```python
from build123d import *

# Parameters (mm, degrees)
KEY1SKETCH_R       = 6.5
KEYPADPAD_DEPTH    = 5
KEY2SKETCH_R       = 6.5
KEYPADPAD001_DEPTH = 5
PIN1SKETCH001_R    = 2
PIN1POCKET_DEPTH   = 10
PIN2SKETCH001_R    = 2
PIN2POCKET_DEPTH   = 10


with BuildPart() as part:
    # key1Sketch → keyPadPad (new body)
    with BuildSketch(Plane.XY):
        with Locations((2, 0)):
            Circle(KEY1SKETCH_R)
    extrude(amount=KEYPADPAD_DEPTH)

    # key2Sketch → keyPadPad001 (join)
    with BuildSketch(Plane.XY.offset(5)):
        with Locations((-2, 0)):
            Circle(KEY2SKETCH_R)
    extrude(amount=KEYPADPAD001_DEPTH)

    # Pin1Sketch001 → Pin1Pocket (cut)
    with BuildSketch(Plane.XY.offset(5)):
        with Locations((1.75, 0)):
            Circle(PIN1SKETCH001_R)
    extrude(amount=-PIN1POCKET_DEPTH, mode=Mode.SUBTRACT)

    # Pin2Sketch001 → Pin2Pocket (cut)
    with BuildSketch(Plane.XY.offset(5)):
        with Locations((3.5, 0)):
            Circle(PIN2SKETCH001_R)
    extrude(amount=-PIN2POCKET_DEPTH, mode=Mode.SUBTRACT)


with BuildPart() as part_1:
    # eccentricKey placement: moved
    add(part.part.moved(Location((0, 0, 10))))


solid = part_1.part
```
The model under review builds one solid part; all positions refer to its coordinate system, in mm. A direction names the side the tool comes from. Round coordinates to 2 decimals unless told otherwise and drop trailing zeros. Order: outer loops, then holes, each group sorted by start corner. A loop starts at its lowest first (then second) coordinate and runs counter-clockwise, first axis right, second up. Notation, with made-up numbers: (87, 58) -> (124, 58) arc R16 cw to (124, 78) -> close; hole circle Ø9 at (31.5, 18.25). An arc over 180 degrees is marked (long way). One line per item, written item: value. Start each with the question number.
Q1. Take a section at A-A (y = 0). Write out the cut boundary in (x, z), and give its area (3 significant figures).
Q2. Machinability: for faces 4 (the face through (6, 0, 15)), 5 (the face through (-2, 0, 20)), 6 (the face through (0.591, -6.345, 12.465)), which of the approach directions +Z, -Z, +X, -X, +Y, -Y give a long, thin tool a straight path to every point of the face, cutting with its end or side? Answer none if there is none.
Q3. Take a section at C-C (x = -2). Write out the cut boundary in (y, z).
Q4. Clearance check with flat-ended pins moving along their axes: pin 1 Ø1 at (y, z) = (-1.5, 13) entering from -X; pin 2 Ø1.5 at (y, z) = (-5, 12) entering from +X; pin 3 Ø1 at (x, y) = (6.5, 3.5) entering from +Z. State where each tip first meets the part, or that it passes through.
Q5. Take a section at D-D (z = 16.75). Write out the cut boundary in (x, y).
Q6. Wall thickness on line 1 (Y direction, x = 1.75, z = 13.3); line 2 (Z direction, x = 7.5, y = 1.5); line 3 (Y direction, x = 3.5, z = 12.75): over which ranges is each line inside the solid? List them lowest first.
Q7. Take a section at B-B (y = -2.5). Write out the cut boundary in (x, z).
Q8. Mouldability with a two-part tool opening along X and no side actions: class faces 1 (the face through (0.999, -5.767, 17.465)), 2 (the face through (-5, 0, 15)), 3 (the face through (-0.25, 0.06, 12.54)) as released by +X, released by -X, zero draft, split by the parting line, or undercut.
Reported:
1. outline: (-8.5, 15) -> (-4.5, 15) -> (-4.5, 10) -> (-0.25, 10) -> (-0.25, 15) -> (4.5, 15) -> (4.5, 20) -> (-8.5, 20) -> close; (5.5, 10) -> (8.5, 10) -> (8.5, 15) -> (5.5, 15) -> close
1. area: 101 mm2
2. face 4: +Z, +X
2. face 5: +Z, +X, -X, +Y, -Y
2. face 6: -Z
3. outline: (-6.5, 15) -> (-5.12, 15) -> (-5.12, 10) -> (5.12, 10) -> (5.12, 15) -> (6.5, 15) -> (6.5, 20) -> (-6.5, 20) -> close
4. pin 1: stops at x = -4.42
4. pin 2: stops at x = 6.92
4. pin 3: stops at z = 15
5. outline: circle Ø13 at (-2, 0)
6. line 1: y = -6.5 to -2, 2 to 6.5
6. line 2: z = 10 to 15
6. line 3: y = -6.32 to -2, 2 to 6.32
7. outline: (-8, 15) -> (-4, 15) -> (-4, 10) -> (8, 10) -> (8, 15) -> (4, 15) -> (4, 20) -> (-8, 20) -> close
8. face 1: split by the parting line
8. face 2: zero draft
8. face 3: undercut
